Read the model definition and answer for the solid it produces. Units are mm, in the model's axes. A direction names the side the tool comes from. Coordinates: 2 decimals unless noted, no trailing zeros. Order: outer loops, then holes, each group sorted by start corner. A loop starts at its lowest first (then second) coordinate and runs counter-clockwise, first axis right, second up. Notation, with made-up numbers: (-39.5, -19) -> (12.5, -19) arc R10 cw to (12.5, -12) -> close; hole circle Ø1 at (80.5, 60). An arc over 180 degrees is marked (long way). Return JSON: item names as keys, results as strings. Group by question number.
```python
from build123d import *

# Parameters (mm, degrees)
F0_R      = 7.5
F1_DEPTH  = 10
F2_W      = 30
F2_H      = 10
F3_DEPTH  = 5
F6_DEPTH  = 30
F7_R      = 10
F8_DEPTH  = 10
F10_DEPTH = 10
F11_R     = 17
F12_DEPTH = 5
F13_DEPTH = 5


with BuildPart() as f1:
    # F0 (on Front) → F1 (new body)
    with BuildSketch(Plane.XZ):
        with BuildLine():
            Line((0, 30), (0, 0))
            Line((0, 0), (30, 0))
            Line((30, 0), (30, 30))
            ThreePointArc((30, 30), (15, 45), (0, 30))
        make_face()
        with Locations((15, 30)):
            Circle(F0_R, mode=Mode.SUBTRACT)
    extrude(amount=F1_DEPTH)

    # F2 (on face) → F3 (join)
    with BuildSketch(Plane(origin=(0, 0, 0), x_dir=(-1, 0, 0), z_dir=(0, 1, 0))):
        with Locations((-15, 5)):
            Rectangle(F2_W, F2_H)
    extrude(amount=F3_DEPTH)


with BuildPart() as f5_1:
    # F5: instance of F1
    add(f1.part.mirror(Plane(origin=(15, 20, 5), x_dir=(-1, 0, 0), z_dir=(0, 1, 0))))


with BuildPart() as f1_1:
    add(f1.part)

    # F6 (add, through all): a face of the model
    f6_faces = [f5_1.part.faces().sort_by_distance(p)[0] for p in [
        (15, 35, 5),
    ]]

    add(f5_1.part)  # F6 merges F5_1
    extrude(f6_faces, amount=F6_DEPTH)

    # F7 (on face) → F8 (cut, through all)
    with BuildSketch(Plane.XY.offset(10)):
        with Locations((15, 20)):
            Circle(F7_R)
    extrude(amount=-F8_DEPTH, mode=Mode.SUBTRACT)

    # F9 (on face) → F10 (join)
    with BuildSketch(Plane.XY.offset(10)):
        with BuildLine():
            Line((0, 6.7712434447), (0, 33.2287565553))
            ThreePointArc((0, 33.2287565553), (-5, 20), (0, 6.7712434447))
        make_face()
        with BuildLine():
            ThreePointArc((30, 6.7712434447), (35, 20), (30, 33.2287565553))
            Line((30, 33.2287565553), (30, 6.7712434447))
        make_face()
    extrude(amount=-F10_DEPTH)

    # F11 (on face) → F12 (join)
    with BuildSketch(Plane(origin=(0, 0, 0), x_dir=(1, 0, 0), z_dir=(0, 0, -1))):
        with Locations((15, -20)):
            Circle(F11_R)
    extrude(amount=F12_DEPTH)

    # F13 (cut, through all): a face of the model
    f13_faces = [f1_1.faces().sort_by_distance(p)[0] for p in [
        (15, 20, 0),
    ]]
    extrude(f13_faces, amount=-F13_DEPTH, mode=Mode.SUBTRACT)


solid = f1_1.part
```
1. Given pin 1 (6 mm diameter, centred on x = 26.5, y = 17.5, fed in from +Z); pin 2 (6 mm diameter, centred on y = 14.5, z = 0, fed in from +X); pin 3 (1 mm diameter, centred on y = -2, z = 10.5, fed in from +X); pin 4 (24 mm diameter, centred on x = 19, z = 33, fed in from +Y), each flat-ended and moving along its own axis, determine where each tip first touches the part or whether it passes through.
2. Find section B-B on z = 13.5. Determine the outline of the cut face in (x, y).
3. Straight lines are drawn through the part: L1, parallel to Y at x = 8.5, z = 14; L2, parallel to Z at x = 21.5, y = 29; L3, parallel to Y at x = 18, z = 1. For each, find the intervals that lie inside material, in ascending order.
4. Find section C-C on y = 20. Determine the outline of the cut face in (x, z).
5. Find section D-D on y = -4.5. Determine the outline of the cut face in (x, z).
6. For a pull along X with two mould halves and no side action, classify faces 4 (the face through (24.54, 23, 2.61)), 5 (the face through (13.37, -4.93, 22.68)), 6 (the face through (0, -3, 11)), 7 (the face through (15, 45, 45)) as released by +X, released by -X, zero draft, split by the parting line, or undercut.
7. Which of the six approach directions +Z, -Z, +X, -X, +Y, -Y give full straight-line access (tool end or side, diameter ignored) to faces 1 (the face through (0, 44, 11)), 2 (the face through (15, 0, 20)), 3 (the face through (30, 44, 11))?
8. Find section A-A on x = 15. Determine the outline of the cut face in (y, z), and give its area (3 significant figures).
Result:
{
 "1": {"pin 1": "z = 10", "pin 2": "x = 34.84", "pin 3": "x = 30", "pin 4": "y = 50"},
 "2": {"outline": "(0, -10) -> (30, -10) -> (30, 0) -> (0, 0) -> close; (0, 40) -> (30, 40) -> (30, 50) -> (0, 50) -> close"},
 "3": {"L1": "-10 to 0, 40 to 50", "L2": "-5 to 10", "L3": "-10 to 10.46, 29.54 to 50"},
 "4": {"outline": "(-5, 0) -> (-2, 0) -> (-2, -5) -> (5, -5) -> (5, 10) -> (-5, 10) -> close; (25, -5) -> (32, -5) -> (32, 0) -> (35, 0) -> (35, 10) -> (25, 10) -> close"},
 "5": {"outline": "(0, 0) -> (30, 0) -> (30, 30) arc R15 ccw to (0, 30) -> close; hole circle Ø15 at (15, 30)"},
 "6": {"face 4": "undercut", "face 5": "undercut", "face 6": "released by -X", "face 7": "split by the parting line"},
 "7": {"face 1": "+Z, -Z, -X, +Y", "face 2": "+Z, +X, -X", "face 3": "+Z, -Z, +X, +Y"},
 "8": {"outline": "(-10, 0) -> (3, 0) -> (3, -5) -> (10, -5) -> (10, 10) -> (0, 10) -> (0, 22.5) -> (-10, 22.5) -> close; (-10, 37.5) -> (0, 37.5) -> (0, 45) -> (-10, 45) -> close; (30, -5) -> (37, -5) -> (37, 0) -> (50, 0) -> (50, 22.5) -> (40, 22.5) -> (40, 10) -> (30, 10) -> close; (40, 37.5) -> (50, 37.5) -> (50, 45) -> (40, 45) -> close", "area": "870 mm^2"}
}
